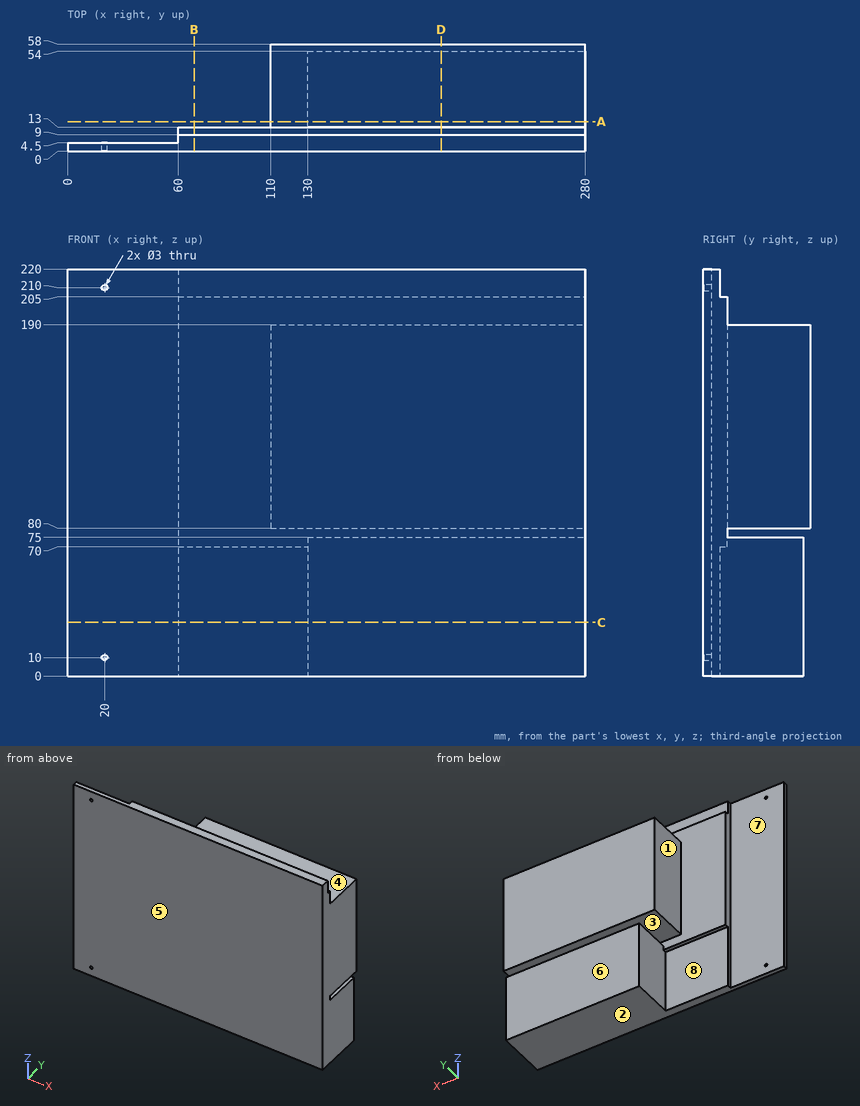
The drawing under review shows one solid part. Ordinate dimensions are in mm from its lowest x, y, z. A direction names the side the tool comes from. Give positions to 0.01 mm unless a question says otherwise; leave off trailing zeros. Order: outer loops, then holes, each group sorted by start corner. A loop starts at its lowest first (then second) coordinate and runs counter-clockwise, first axis right, second up. Notation, with made-up numbers: M -3.5,80 L 16.5,80 A24 cw 16.5,111 Z; hole C -9,70.5 d9. An arc over 180 degrees is marked long. Answer in a Markdown table with one row per item. Add a question column.
1. Add section A-A on y = 16. State the section outline as (x, z) points, plus the area to 4 significant figures.
2. For pin 1 Ø6 at (y, z) = (27.5, 48) entering from -X; pin 2 Ø22.5 at (x, y) = (185.5, 42.5) entering from +Z; pin 3 Ø12 at (y, z) = (25, 162.5) entering from -X; pin 4 Ø2.5 at (x, z) = (20, 210) entering from +Y, all flat-tipped, find the tip position at first contact; note any pin that passes through.
3. Add section D-D on x = 202. State the section outline as (y, z) points.
4. Add section B-B on x = 68.5. State the section outline as (y, z) points.
5. To check wall thickness, follow line 1 along Z through (x, y) = (20, 2); line 2 along Z through (x, y) = (239.5, 25); line 3 along X through (y, z) = (2.35, 210). State the ranges of each line that lie inside material, in increasing order.
6. Machinability: for the marked faces 5, 6, 7 and 8, which of the approach directions +Z, -Z, +X, -X, +Y, -Y give a long, thin tool a straight path to every point of the face, cutting with its end or side? Answer none if there is none.
7. Add section C-C on z = 29. State the section outline as (x, y) points, plus the area to 3 significant figures.
8. Mouldability with a two-part tool opening along Z and no side actions: class the marked faces 1, 2, 3 and 4 as released by +Z, released by -Z, zero draft, split by the parting line, or undercut.
The answers:
| question | item | result |
|---|---|---|
| 1 | outline | M 110,80 L 280,80 L 280,190 L 110,190 Z; M 130,0 L 280,0 L 280,75 L 130,75 Z |
| 1 | area | 29,950 mm2 |
| 2 | pin 1 | x = 130 |
| 2 | pin 2 | z = 190 |
| 2 | pin 3 | x = 110 |
| 2 | pin 4 | through |
| 3 | outline | M 0,0 L 54,0 L 54,75 L 13,75 L 13,80 L 58,80 L 58,190 L 13,190 L 13,205 L 9,205 L 9,220 L 0,220 Z |
| 4 | outline | M 0,0 L 9,0 L 9,70 L 13,70 L 13,205 L 9,205 L 9,220 L 0,220 Z |
| 5 | line 1 | 0 to 8.5, 11.5 to 208.5, 211.5 to 220 |
| 5 | line 2 | 0 to 75, 80 to 190 |
| 5 | line 3 | 0 to 18.5, 21.5 to 280 |
| 6 | face 5 | +Z, -Z, +X, -X, -Y |
| 6 | face 6 | -Z, +X, -X, +Y |
| 6 | face 7 | +Z, -Z, -X, +Y |
| 6 | face 8 | -Z, -X, +Y |
| 7 | outline | M 0,0 L 280,0 L 280,54 L 130,54 L 130,9 L 60,9 L 60,4.5 L 0,4.5 Z |
| 7 | area | 9,000 mm2 |
| 8 | face 1 | zero draft |
| 8 | face 2 | released by -Z |
| 8 | face 3 | undercut |
| 8 | face 4 | released by +Z |
